Check sheet for the modelled part. Datum: model origin and axes. Units: mm. A direction names the side the tool comes from. Round coordinates to 2 decimals unless told otherwise and drop trailing zeros. Write each loop counter-clockwise with the first axis right and the second up, starting at its lowest first coordinate (ties: lowest second). Pieces come first, ordered by that corner, then holes. Notation, with made-up numbers: M 43,77 L 62,77 A19 ccw 62,84 Z; hole C -15,-11 d4. An arc over 180 degrees is marked long. One line per item, written item: value.
from build123d import *

# Parameters (mm, degrees)
SKETCH1_W           = 500
SKETCH1_H           = 25
BOSS_EXTRUDE1_DEPTH = 25
SKETCH2_R           = 5
CUT_EXTRUDE1_DEPTH  = 25
SKETCH5_W           = 20.75
SKETCH5_H           = 5
CUT_EXTRUDE2_DEPTH  = 25


with BuildPart() as part:
    # Sketch1 → Boss-Extrude1 (new body)
    with BuildSketch(Plane(origin=(0, 0, 0), x_dir=(1, 0, 0), z_dir=(0, 1, 0))):
        Rectangle(SKETCH1_W, SKETCH1_H)
    extrude(amount=BOSS_EXTRUDE1_DEPTH)

    # Sketch2 → Cut-Extrude1 (cut)
    with BuildSketch(Plane.XY.offset(12.5)):
        with Locations((-235, 12.5)):
            Circle(SKETCH2_R)
        with Locations((-50, 12.5)):
            Circle(SKETCH2_R)
    extrude(amount=-CUT_EXTRUDE1_DEPTH, mode=Mode.SUBTRACT)

    # Sketch5 → Cut-Extrude2 (cut)
    with BuildSketch(Plane(origin=(0, 25, 0), x_dir=(1, 0, 0), z_dir=(0, 1, 0))):
        with Locations((239.670802425, 0)):
            Rectangle(SKETCH5_W, SKETCH5_H)
    extrude(amount=-CUT_EXTRUDE2_DEPTH, mode=Mode.SUBTRACT)


solid = part.part
Q1. Draft check along X on faces 3 (the flat face through (240, 13, -2.5)), 4 (the flat face through (250, 12, -7)), 5 (the cylindrical face through (-53.685, 15.879, 0.175)), 6 (the cylindrical face through (-230.23, 14, 0.18)). Enter one of: pulls with the +X half, pulls with the -X half, needs draft (parallel to the pull), parting line crosses it, or undercut.
Completed:
face 3: needs draft
face 4: pulls with the +X half
face 5: undercut
face 6: undercut
Q2. Access from +Z, -Z, +X, -X, +Y, -Y to the whole of each face (thin tool, end or side, straight path). Record for faces 1 (the flat face through (-3, 25, 0)), 2 (the flat face through (240, 13, 2.5)).
Completed:
face 1: +Z, -Z, +X, -X, +Y
face 2: +X, +Y, -Y
Q3. Sectioned sample at A-A on x = -235. Enter the section's corners in (y, z).
Completed:
outline: M 0,-12.5 L 7.5,-12.5 L 7.5,12.5 L 0,12.5 Z; M 17.5,-12.5 L 25,-12.5 L 25,12.5 L 17.5,12.5 Z
Q4. Depth check by flat-ended pin: P1, Ø8, axis at x = -155, z = 7.5, coming from the -Y side; P2, Ø4, axis at y = 7.5, z = 0, coming from the +X side; P3, Ø8, axis at x = -235, y = 12.5, coming from the +Z side. Enter the tip coordinate at first touch or a pass-through.
Completed:
P1: y = 0
P2: x = 229.3
P3: through
Q5. Scan line: line 1 (Y direction, x = -235, z = 0.25). Record every from-to range of solid material in increasing order. Write a range as [from, to].
Completed:
line 1: [0, 7.5], [17.5, 25]
